Verification items for the finished model (mm, model axes). Coordinates: 2 decimals unless noted, no trailing zeros. Order: outer loops, then holes, each group sorted by start corner. A loop starts at its lowest first (then second) coordinate and runs counter-clockwise, first axis right, second up. Notation, with made-up numbers: (89.25, 47) - (109.25, 47) arc R26 cw to (109.25, 61) - close; hole circle Ø7 at (62.25, -40). An arc over 180 degrees is marked (long way). Answer as CSV lines item,"result". Start each with the question number.
1. Section check A-A (x = -2.5). Record the cut outline in (y, z).
2. Section check C-C (z = 18.5). Record the cut outline in (x, y), and give its area (3 significant figures).
3. Go/stop test with flat-tipped pins: pin 1 (3 mm diameter, centred on x = -3, y = 2, fed in from +Z); pin 2 (2 mm diameter, centred on x = -2, y = 0.5, fed in from -Z); pin 3 (1.2 mm diameter, centred on x = -2, z = 2.5, fed in from +Y). Record where each tip stops, or that it passes through.
4. Material ranges on L1, parallel to X at y = 0.7, z = 92; L2, parallel to Z at x = -2, y = 1.85, recorded low to high. Write a range as [from, to].
5. Section check B-B (y = 2.55). Record the cut outline in (x, z), and give its area (3 significant figures).
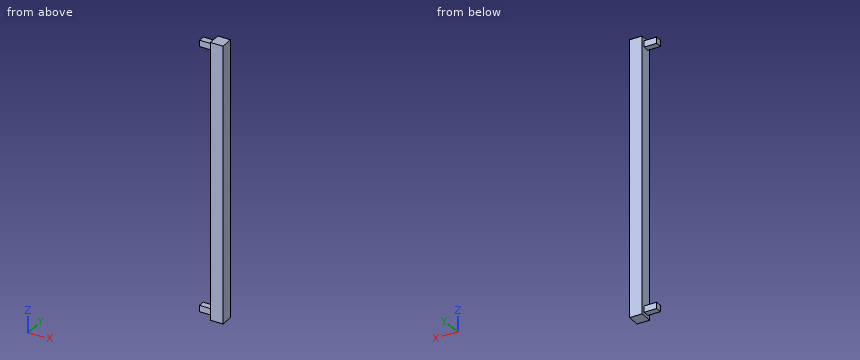
from build123d import *

# Parameters (mm, degrees)
SKETCH1_W           = 5
SKETCH1_H           = 5
BOSS_EXTRUDE1_DEPTH = 110
SKETCH2_W           = 2.5
SKETCH2_H           = 2.5
BOSS_EXTRUDE2_DEPTH = 5


with BuildPart() as part:
    # Sketch1 → Boss-Extrude1 (new body)
    with BuildSketch(Plane.XY):
        with Locations((2.5, 2.5)):
            Rectangle(SKETCH1_W, SKETCH1_H)
    extrude(amount=BOSS_EXTRUDE1_DEPTH)

    # Sketch2 → Boss-Extrude2 (add)
    with BuildSketch(Plane.ZY):
        with Locations((2.5, 2.5)):
            Rectangle(SKETCH2_W, SKETCH2_H)
        with Locations((107.5, 2.5)):
            Rectangle(SKETCH2_W, SKETCH2_H)
    extrude(amount=BOSS_EXTRUDE2_DEPTH)


solid = part.part
Evaluation:
1,outline,"(1.25, 1.25) - (3.75, 1.25) - (3.75, 3.75) - (1.25, 3.75) - close; (1.25, 106.25) - (3.75, 106.25) - (3.75, 108.75) - (1.25, 108.75) - close"
2,outline,"(0, 0) - (5, 0) - (5, 5) - (0, 5) - close"
2,area,"25.0 mm²"
3,pin 1,"stops at z = 108.75"
3,pin 2,"stops at z = 1.25"
3,pin 3,"stops at y = 3.75"
4,L1,"x = [0, 5]"
4,L2,"z = [1.25, 3.75], [106.25, 108.75]"
5,outline,"(-5, 1.25) - (0, 1.25) - (0, 0) - (5, 0) - (5, 110) - (0, 110) - (0, 108.75) - (-5, 108.75) - (-5, 106.25) - (0, 106.25) - (0, 3.75) - (-5, 3.75) - close"
5,area,"575 mm²"
